Work out the finished part from the listing and answer in its coordinate system (mm). A direction names the side the tool comes from. Give positions to 0.01 mm unless a question says otherwise; leave off trailing zeros. Order: outer loops, then holes, each group sorted by start corner. A loop starts at its lowest first (then second) coordinate and runs counter-clockwise, first axis right, second up. Notation, with made-up numbers: M 32,21.5 L 72,21.5 A27 cw 72,39.5 Z; hole C 7,4 d4. An arc over 180 degrees is marked long. One line per item, written item: value.
from build123d import *

# Parameters (mm, degrees)
SKETCH_1_R           = 23.5
SKETCH_1_R_2         = 22
EXTRUDE_1_DEPTH      = 20
EXTRUDE_1_DEPTH_BACK = 10
SKETCH_3_R           = 25
SKETCH_3_R_2         = 23
EXTRUDE_2_DEPTH      = 10
EXTRUDE_2_DEPTH_BACK = 10
SKETCH_4_R           = 25
SKETCH_4_R_2         = 23
SKETCH_5_R           = 2.75
EXTRUDE_3_DEPTH      = 5


with BuildPart() as part:
    # Sweep 1: sweep along a path in Sketch 2
    with BuildLine(Plane.XY) as sweep_1_path:
        Line((0, 0), (0, 20))
        ThreePointArc((0, 20), (-19.464587543, 64.236640209), (-65.229344565, 79.771681886))
        Line((-65.229344565, 79.771681886), (-85.153238527, 78.028567031))
    # Sketch 1 → Sweep 1 (sweep)
    with BuildSketch(Plane(origin=(0, 0, 0), x_dir=(1, 0, 0), z_dir=(0, 1, 0))):
        Circle(SKETCH_1_R)
        Circle(SKETCH_1_R_2, mode=Mode.SUBTRACT)
    sweep(path=sweep_1_path.line)

    # Sketch 4 → Extrude 2 (add, two sides: drawn at the far end of the back side and taken through both)
    with BuildSketch(Plane(origin=(-77.731644776, -6.800637715, 0), x_dir=(0, 0, 1), z_dir=(-0.9961946980917464, -0.08715574274764801, 0)).offset(-EXTRUDE_2_DEPTH_BACK)):
        with Locations(Location((0, 85.153238527, 0), (0, 0, 270))):
            Circle(SKETCH_4_R)
        with Locations(Location((0, 85.153238527, 0), (0, 0, 270))):
            Circle(SKETCH_4_R_2, mode=Mode.SUBTRACT)
    extrude(amount=EXTRUDE_2_DEPTH + EXTRUDE_2_DEPTH_BACK)


with BuildPart() as body_2:
    # Sketch 3 → Extrude 1 (new, two sides: drawn at the far end of the back side and taken through both)
    with BuildSketch(Plane.XZ.offset(-EXTRUDE_1_DEPTH_BACK)):
        with Locations(Location((0, 0, 0), (0, 0, 270))):
            Circle(SKETCH_3_R)
        with Locations(Location((0, 0, 0), (0, 0, 270))):
            Circle(SKETCH_3_R_2, mode=Mode.SUBTRACT)
    extrude(amount=EXTRUDE_1_DEPTH + EXTRUDE_1_DEPTH_BACK)


    add(part.part)  # Extrude 3 merges part
    # Sketch 5 → Extrude 3 (add)
    with BuildSketch(Plane(origin=(0, 0, 0), x_dir=(-1, 0, 0), z_dir=(0, -1, 0))):
        with BuildLine():
            Line((-44, 15), (-20, 15))
            ThreePointArc((-20, 15), (-25, 0), (-20, -15))
            Line((-20, -15), (-44, -15))
            Line((-44, -15), (-44, 15))
        make_face()
        with Locations(Location((-36, 0, 0), (0, 0, 90))):
            Circle(SKETCH_5_R, mode=Mode.SUBTRACT)
    extrude(amount=-EXTRUDE_3_DEPTH)


solid = body_2.part
(1) Section B-B, the plane y = -9 is taken. Give the vertices of the cut face in (x, z).
Findings:
outline: C 0,0 d50; hole C 0,0 d46
(2) Determine the mould class of faces 4 (the cylindrical face through (-70.01, 76.28, -23.3)), 5 (the flat face through (-12, 0, 19)), 6 (the flat face through (32, 0, 0)) for opening direction Z: pulls with the +Z half, pulls with the -Z half, needs draft (parallel to the pull), parting line crosses it, or undercut.
Findings:
face 4: parting line crosses it
face 5: undercut
face 6: needs draft
(3) Given P1, Ø5.5, axis at x = 28, y = 3.5, coming from the -Z side; P2, Ø5, axis at y = -5, z = -14, coming from the -X side; P3, Ø10, axis at y = 69, z = -7.5, coming from the +X side; P4, Ø7, axis at x = 26, z = -6.5, coming from the -Y side, each flat-ended and moving along its own axis, determine where each tip first touches the part or whether it passes through.
Findings:
P1: stops at z = -15
P2: stops at x = -22.2
P3: stops at x = 9.93
P4: stops at y = -20
(4) Section A-A, the plane x = 36 is taken. Give the vertices of the cut face in (y, z), then the cut area to 4 significant figures.
Findings:
outline: M 0,-15 L 5,-15 L 5,-2.75 L 0,-2.75 Z; M 0,2.75 L 5,2.75 L 5,15 L 0,15 Z
area: 122.5 mm^2
(5) Section D-D, the plane z = 0 is taken. Give the number of separate pieces and of enclosed holes in the cut face, then the cut area to 3 significant figures.
Findings:
separate pieces: 3
enclosed holes: 0
area: 666 mm^2
(6) Which of the six approach directions +Z, -Z, +X, -X, +Y, -Y give full straight-line access (tool end or side, diameter ignored) to faces 1 (the cylindrical face through (38.727, 2.465, 0.358)), 2 (the flat face through (-17, 10, 17)), 3 (the cylindrical face through (-4.769, 10.14, 21.477))?
Findings:
face 1: +Y, -Y
face 2: none
face 3: -Y
(7) Find the intervals of material crossed by probe 1 along X at (y, z) = (3.7, 0); probe 2 along X at (y, z) = (-11.5, 0.5) (3 decimals); probe 3 along X at (y, z) = (13.5, 0), in increasing order. Write a range as from..to.
Findings:
probe 1: x = -25..-22, 22..33.25, 38.75..44
probe 2: x = -24.995..-22.995, 22.995..24.995
probe 3: x = -23.5..-22, 22..23.5
